Could you check a few things on this model? Use its own coordinates, in mm. Face numbers are marked on the shaded views. A direction names the side the tool comes from. Coordinates: 2 decimals unless noted, no trailing zeros. Loops run counter-clockwise (first coordinate to the right, second up) from the corner with the lowest first, then second, coordinate; pieces in that order, holes last.
1) If I drill on line 1 along Y through (x, z) = (41, 16); line 2 along X through (y, z) = (-8.75, 18), over which ranges is the centre line in solid material (lowest first)?
2) Imagine slicing it at A-A on z = 23. Please give me the cut outline in (x, y).
3) For the marked faces 4, 5, 6 and 7, which set-ups out of +Z, -Z, +X, -X, +Y, -Y let a thin tool reach every point of the face, with its end or its side?
4) Imagine slicing it at D-D on y = -11. Please give me the cut outline in (x, z), plus the area to 3 significant figures.
5) Thinking about a two-plate mould opening in X: for the marked faces 1, 2 and 3, which applies, released by +X, released by -X, zero draft, split by the parting line, or undercut?
6) Will these pins go through, and if not, where does the flat tip stop? P1, Ø12, axis at y = -19.5, z = 7.5, coming from the +X side; P2, Ø7, axis at x = 46, y = -17.5, coming from the +Z side; P3, Ø1, axis at y = -10, z = 6.5, coming from the -X side.
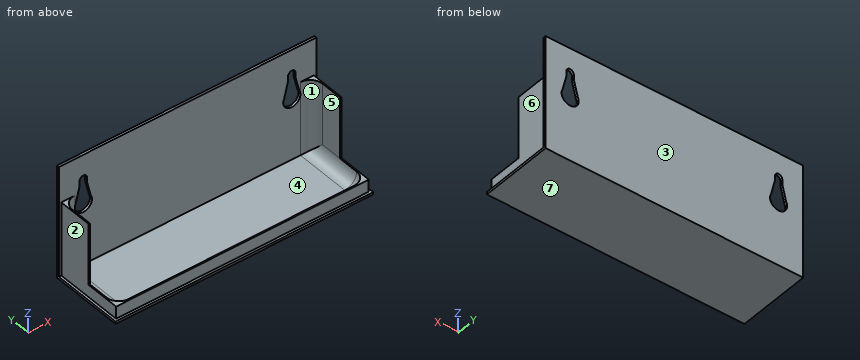
```python
from build123d import *

# Parameters (mm, degrees)
F0_W     = 102
F0_H     = 27.5
F1_DEPTH = 1
F2_DEPTH = 5
F4_DEPTH = 25
F6_DEPTH = 15
F8_DEPTH = 1
F9_R     = 4.99999
F10_R    = 4.99999


# Not quite as in the source:
# - a fillet or chamfer is up to 0.001 mm smaller than in the source, because OpenCascade refuses the exact size
# - a feature names something its author has since deleted; it is built from what else it names


with BuildPart() as f1:
    # F0 (on Top) → F1 (new body)
    with BuildSketch(Plane.XY):
        with Locations((52.5, -14.75)):
            Rectangle(F0_W, F0_H)
        Polygon((1.5, -1), (1, -1), (1, -29), (104, -29), (104, -1), (103.5, -1), (103.5, -28.5), (1.5, -28.5), align=None)
        Polygon((1, -1), (0, -1), (0, -30), (105, -30), (105, -1), (104, -1), (104, -29), (1, -29), align=None)
        Polygon((105, 0), (0, 0), (0, -1), (1, -1), (1.5, -1), (103.5, -1), (104, -1), (105, -1), align=None)
    extrude(amount=-F1_DEPTH)

    # F0 (on Top) → F2 (join)
    with BuildSketch(Plane.XY):
        Polygon((105, 0), (0, 0), (0, -1), (1, -1), (1.5, -1), (103.5, -1), (104, -1), (105, -1), align=None)
        Polygon((1.5, -1), (1, -1), (1, -29), (104, -29), (104, -1), (103.5, -1), (103.5, -28.5), (1.5, -28.5), align=None)
    extrude(amount=F2_DEPTH)

    # F3 (on face) → F4 (join)
    with BuildSketch(Plane.XY.offset(5)):
        Polygon((1, -1), (1, -15), (1.5, -15), (1.5, -1), (103.5, -1), (103.5, -15), (104, -15), (104, -1), (105, -1), (105, 0), (0, 0), (0, -1), align=None)
    extrude(amount=F4_DEPTH)

    # F5 (on face) → F6 (join)
    with BuildSketch(Plane.XY.offset(30)):
        Polygon((1.5, -1), (103.5, -1), (104, -1), (105, -1), (105, 0), (0, 0), (0, -1), (1, -1), align=None)
    extrude(amount=F6_DEPTH)

    # F7 (on face) → F8 (cut, through all)
    with BuildSketch(Plane.XZ.offset(1)):
        with BuildLine():
            Line((13.5, 25), (6.5, 25))
            ThreePointArc((6.5, 25), (10, 21.5), (13.5, 25))
        make_face()
        with BuildLine():
            ThreePointArc((6.9117647059, 26.6470588235), (6.6045012495, 25.8488746876), (6.5, 25))
            Line((6.5, 25), (6.9117647059, 26.6470588235))
        make_face()
        with BuildLine():
            Line((6.9117647059, 26.6470588235), (6.5, 25))
            Line((6.5, 25), (13.5, 25))
            Line((13.5, 25), (13.0882352941, 26.6470588235))
            ThreePointArc((13.0882352941, 26.6470588235), (10, 28.5), (6.9117647059, 26.6470588235))
        make_face()
        with BuildLine():
            Line((13.0882352941, 26.6470588235), (13.5, 25))
            ThreePointArc((13.5, 25), (13.3954987505, 25.8488746876), (13.0882352941, 26.6470588235))
        make_face()
        with BuildLine():
            Line((8.5, 33), (6.9117647059, 26.6470588235))
            ThreePointArc((6.9117647059, 26.6470588235), (10, 28.5), (13.0882352941, 26.6470588235))
            Line((13.0882352941, 26.6470588235), (11.5, 33))
            ThreePointArc((11.5, 33), (10, 31.5), (8.5, 33))
        make_face()
        with BuildLine():
            ThreePointArc((8.8819660113, 34), (8.5987414616, 33.5352331347), (8.5, 33))
            ThreePointArc((8.5, 33), (10, 31.5), (11.5, 33))
            ThreePointArc((11.5, 33), (11.4012585384, 33.5352331347), (11.1180339887, 34))
            ThreePointArc((11.1180339887, 34), (10, 33.5), (8.8819660113, 34))
        make_face()
        with BuildLine():
            Line((8.5, 35), (8.5, 33))
            ThreePointArc((8.5, 33), (8.5987414616, 33.5352331347), (8.8819660113, 34))
            ThreePointArc((8.8819660113, 34), (8.5987414616, 34.4647668653), (8.5, 35))
        make_face()
        with BuildLine():
            ThreePointArc((11.1180339887, 34), (11.4012585384, 33.5352331347), (11.5, 33))
            Line((11.5, 33), (11.5, 35))
            ThreePointArc((11.5, 35), (11.4012585384, 34.4647668653), (11.1180339887, 34))
        make_face()
        with BuildLine():
            ThreePointArc((8.5, 35), (8.5987414616, 34.4647668653), (8.8819660113, 34))
            ThreePointArc((8.8819660113, 34), (10, 34.5), (11.1180339887, 34))
            ThreePointArc((11.1180339887, 34), (11.4012585384, 34.4647668653), (11.5, 35))
            Line((11.5, 35), (8.5, 35))
        make_face()
        with BuildLine():
            ThreePointArc((11.5, 35), (10, 36.5), (8.5, 35))
            Line((8.5, 35), (11.5, 35))
        make_face()
        with BuildLine():
            Line((91.9117647059, 26.6470588235), (91.5, 25))
            ThreePointArc((91.5, 25), (95, 21.5), (98.5, 25))
            Line((98.5, 25), (98.0882352941, 26.6470588235))
            ThreePointArc((98.0882352941, 26.6470588235), (95, 28.5), (91.9117647059, 26.6470588235))
        make_face()
        with BuildLine():
            ThreePointArc((91.9117647059, 26.6470588235), (91.6045012495, 25.8488746876), (91.5, 25))
            Line((91.5, 25), (91.9117647059, 26.6470588235))
        make_face()
        with BuildLine():
            Line((98.0882352941, 26.6470588235), (98.5, 25))
            ThreePointArc((98.5, 25), (98.3954987505, 25.8488746876), (98.0882352941, 26.6470588235))
        make_face()
        with BuildLine():
            Line((93.5, 33), (91.9117647059, 26.6470588235))
            ThreePointArc((91.9117647059, 26.6470588235), (95, 28.5), (98.0882352941, 26.6470588235))
            Line((98.0882352941, 26.6470588235), (96.5, 33))
            ThreePointArc((96.5, 33), (95, 31.5), (93.5, 33))
        make_face()
        with BuildLine():
            ThreePointArc((93.8819660113, 34), (93.5987414616, 33.5352331347), (93.5, 33))
            ThreePointArc((93.5, 33), (95, 31.5), (96.5, 33))
            ThreePointArc((96.5, 33), (96.4012585384, 33.5352331347), (96.1180339887, 34))
            ThreePointArc((96.1180339887, 34), (95, 33.5), (93.8819660113, 34))
        make_face()
        with BuildLine():
            Line((93.5, 35), (93.5, 33))
            ThreePointArc((93.5, 33), (93.5987414616, 33.5352331347), (93.8819660113, 34))
            ThreePointArc((93.8819660113, 34), (93.5987414616, 34.4647668653), (93.5, 35))
        make_face()
        with BuildLine():
            ThreePointArc((96.1180339887, 34), (96.4012585384, 33.5352331347), (96.5, 33))
            Line((96.5, 33), (96.5, 35))
            ThreePointArc((96.5, 35), (96.4012585384, 34.4647668653), (96.1180339887, 34))
        make_face()
        with BuildLine():
            ThreePointArc((93.5, 35), (93.5987414616, 34.4647668653), (93.8819660113, 34))
            ThreePointArc((93.8819660113, 34), (95, 34.5), (96.1180339887, 34))
            ThreePointArc((96.1180339887, 34), (96.4012585384, 34.4647668653), (96.5, 35))
            ThreePointArc((96.5, 35), (95, 36.5), (93.5, 35))
        make_face()
        with BuildLine():
            ThreePointArc((11.1180339887, 34), (10, 34.5), (8.8819660113, 34))
            ThreePointArc((8.8819660113, 34), (10, 33.5), (11.1180339887, 34))
        make_face()
        with BuildLine():
            ThreePointArc((96.1180339887, 34), (95, 34.5), (93.8819660113, 34))
            ThreePointArc((93.8819660113, 34), (95, 33.5), (96.1180339887, 34))
        make_face()
    extrude(amount=-F8_DEPTH, mode=Mode.SUBTRACT)

    # F9 (radius 5 in the source; OpenCascade refuses exactly that, so slightly less here)
    f9_edges = [f1.edges().sort_by_distance(p)[0] for p in [
        (1.5, -14.75, 0),
        (103.5, -14.75, 0),
        (103.5, -1, 15),
        (1.5, -1, 15),
    ]]
    fillet(f9_edges, radius=F9_R)

    # F10 (radius 5 in the source; OpenCascade refuses exactly that, so slightly less here)
    f10_edges = [f1.edges().sort_by_distance(p)[0] for p in [
        (52.5, -28.5, 0),
    ]]
    fillet(f10_edges, radius=F10_R)


solid = f1.part
```
Filled in:
1. line 1: y = -1 to 0
1. line 2: x = 1 to 1.5, 103.5 to 104
2. outline: (0, -1) - (1, -1) - (1, -15) - (1.5, -15) - (1.5, -6) arc R5 cw to (6.5, -1) - (7.13, -1) - (7.13, 0) - (0, 0) - close; (12.87, -1) - (92.13, -1) - (92.13, 0) - (12.87, 0) - close; (97.87, -1) - (98.5, -1) arc R5 cw to (103.5, -6) - (103.5, -15) - (104, -15) - (104, -1) - (105, -1) - (105, 0) - (97.87, 0) - close
3. face 4: +Z
3. face 5: +Z, -Y
3. face 6: +Z, +X, -Y
3. face 7: -Z, +X, -X, +Y, -Y
4. outline: (0, -1) - (105, -1) - (105, 0) - (104, 0) - (104, 30) - (103.5, 30) - (103.5, 5) arc R5 cw to (98.5, 0) - (6.5, 0) arc R5 cw to (1.5, 5) - (1.5, 30) - (1, 30) - (1, 0) - (0, 0) - close
4. area: 146 mm2
5. face 1: undercut
5. face 2: released by -X
5. face 3: zero draft
6. P1: stops at x = 104
6. P2: stops at z = 0
6. P3: stops at x = 1
